```python
from build123d import *

# Parameters (mm, degrees)
F0_W     = 304.8
F0_H     = 304.8
F1_DEPTH = 19.05
F2_W     = 25.4
F2_H     = 15.24
F3_DEPTH = 43.18
F4_W     = 25.4
F4_H     = 15.24
F5_DEPTH = 43.18
F6_W     = 25.4
F6_H     = 15.24
F7_DEPTH = 43.18
F8_W     = 25.4
F8_H     = 15.24
F9_DEPTH = 43.18


with BuildPart() as f1:
    # F0 (on Top) → F1 (new body)
    with BuildSketch(Plane.XY):
        with Locations((-152.4, 152.4)):
            Rectangle(F0_W, F0_H)
    extrude(amount=F1_DEPTH)

    # F2 (on face) → F3 (cut)
    with BuildSketch(Plane.XZ):
        with Locations((-228.6, 11.43)):
            Rectangle(F2_W, F2_H)
    extrude(amount=-F3_DEPTH, mode=Mode.SUBTRACT)

    # F4 (on face) → F5 (cut)
    with BuildSketch(Plane.XZ):
        with Locations((-74.026464, 11.43)):
            Rectangle(F4_W, F4_H)
    extrude(amount=-F5_DEPTH, mode=Mode.SUBTRACT)

    # F6 (on face) → F7 (cut)
    with BuildSketch(Plane(origin=(0, 304.8, 0), x_dir=(-1, 0, 0), z_dir=(0, 1, 0))):
        with Locations((139.7, 11.43)):
            Rectangle(F6_W, F6_H)
    extrude(amount=-F7_DEPTH, mode=Mode.SUBTRACT)

    # F8 (on face) → F9 (cut)
    with BuildSketch(Plane.YZ):
        with Locations((145.6436, 11.43)):
            Rectangle(F8_W, F8_H)
    extrude(amount=-F9_DEPTH, mode=Mode.SUBTRACT)


solid = f1.part
```
Source: CAD feature listing. Evaluate the final solid. Frame: model axes, mm. A direction names the side the tool comes from. Give positions to 0.01 mm unless a question says otherwise; leave off trailing zeros. Loops run counter-clockwise (first coordinate to the right, second up) from the corner with the lowest first, then second, coordinate; pieces in that order, holes last. Notation, with made-up numbers: (17.25, -4) - (76.25, -4) arc R7 cw to (76.25, 2) - close; hole circle Ø3 at (33, -7). An arc over 180 degrees is marked (long way). Use CSV: the item, a comma, the result in double quotes.
1) Line query: line 1 (X direction, y = 43, z = 17.5); line 2 (X direction, y = 275, z = 8); line 3 (Z direction, x = -131.5, y = 287). Output: solid intervals per line, ascending.
Worked out:
line 1,"x = -304.8 to -241.3, -215.9 to -86.73, -61.33 to 0"
line 2,"x = -304.8 to -152.4, -127 to 0"
line 3,"z = 0 to 3.81"
2) Cut plane B-B (z = 16). Output: boundary loops of the cut face in (x, y), and give its area (3 significant figures).
Worked out:
outline,"(-304.8, 0) - (-241.3, 0) - (-241.3, 43.18) - (-215.9, 43.18) - (-215.9, 0) - (-86.73, 0) - (-86.73, 43.18) - (-61.33, 43.18) - (-61.33, 0) - (0, 0) - (0, 132.94) - (-43.18, 132.94) - (-43.18, 158.34) - (0, 158.34) - (0, 304.8) - (-127, 304.8) - (-127, 261.62) - (-152.4, 261.62) - (-152.4, 304.8) - (-304.8, 304.8) - close"
area,"88,500 mm^2"
3) Mould query, pull axis X, two halves, no side actions, for faces 6 (the flat face through (-61.326, 21, 11)), 7 (the flat face through (-155, 0, 9)), 8 (the flat face through (0, 150, 3)). Classes: +X half, -X half, draft (parallel to the pull), parting line (faces both ways), or undercut.
Worked out:
face 6,"undercut"
face 7,"draft"
face 8,"+X half"
4) Pin query (flat end, axial travel): P1, Ø12.5, axis at x = -137.5, y = 291.5, coming from the +Z side; P2, Ø2, axis at y = 150, z = 13.5, coming from the +X side; P3, Ø5, axis at x = -66, z = 11.5, coming from the -Y side. Return the tip coordinate at first contact, or that it passes through.
Worked out:
P1,"stops at z = 3.81"
P2,"stops at x = -43.18"
P3,"stops at y = 43.18"
5) Cut plane A-A (y = 35.5). Output: boundary loops of the cut face in (x, z).
Worked out:
outline,"(-304.8, 0) - (0, 0) - (0, 19.05) - (-61.33, 19.05) - (-61.33, 3.81) - (-86.73, 3.81) - (-86.73, 19.05) - (-215.9, 19.05) - (-215.9, 3.81) - (-241.3, 3.81) - (-241.3, 19.05) - (-304.8, 19.05) - close"
6) Set-up query: faces 1 (the flat face through (-43.18, 145, 12)), 2 (the flat face through (-140, 261.62, 12)), 3 (the flat face through (-155, 155, 0)), 4 (the flat face through (-241.3, 21, 11)), 5 (the flat face through (-304.8, 150, 9)). Return all of +Z, -Z, +X, -X, +Y, -Y with unobstructed straight access to the full face (end or side cutting, diameter ignored); none if empty.
Worked out:
face 1,"+Z, +X"
face 2,"+Z, +Y"
face 3,"-Z, +X, -X, +Y, -Y"
face 4,"+Z, -Y"
face 5,"+Z, -Z, -X, +Y, -Y"
7) Cut plane C-C (x = -148). Output: boundary loops of the cut face in (y, z).
Worked out:
outline,"(0, 0) - (304.8, 0) - (304.8, 3.81) - (261.62, 3.81) - (261.62, 19.05) - (0, 19.05) - close"
